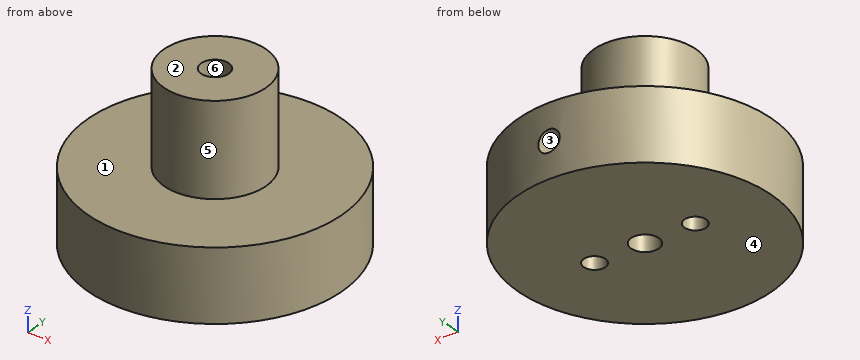
```python
from build123d import *

# Parameters (mm, degrees)
SKETCH1_R                 = 15.8115
BOSS_EXTRUDE1_DEPTH       = 25.4
SKETCH2_OUTSIDE_W         = 43.91
SKETCH2_OUTSIDE_H         = 43.91
SKETCH2_OUTSIDE_R         = 6.35
CUT_EXTRUDE1_DEPTH        = 16.51
F_8_32_TAPPED_HOLE1_D     = 3.4544
F_6_32_TAPPED_HOLE2_D     = 2.7051
F_6_32_TAPPED_HOLE2_DEPTH = 6.858
F_6_32_TAPPED_HOLE2_TIP   = 0.81269403
F_6_32_TAPPED_HOLE3_D     = 2.7051
F_6_32_TAPPED_HOLE3_DEPTH = 6.096
F_6_32_TAPPED_HOLE3_TIP   = 0.81269403
SKETCH9_R                 = 6.35
CUT_EXTRUDE3_DEPTH        = 5.08


with BuildPart() as part:
    # Sketch1 → Boss-Extrude1 (new body)
    with BuildSketch(Plane.XY):
        Circle(SKETCH1_R)
    extrude(amount=BOSS_EXTRUDE1_DEPTH)

    # Sketch2 outside → Cut-Extrude1 (cut)
    with BuildSketch(Plane.XY.offset(25.4)):
        Rectangle(SKETCH2_OUTSIDE_W, SKETCH2_OUTSIDE_H)
        Circle(SKETCH2_OUTSIDE_R, mode=Mode.SUBTRACT)
    extrude(amount=-CUT_EXTRUDE1_DEPTH, mode=Mode.SUBTRACT)

    # #8-32 Tapped Hole1 (through all)
    with Locations(Plane.XY.offset(25.4)):
        with Locations((0, 0)):
            Hole(F_8_32_TAPPED_HOLE1_D / 2)

    # #6-32 Tapped Hole2
    with Locations(Plane(origin=(0, 0, 0), x_dir=(-1, 0, 0), z_dir=(0, 0, -1))):
        with Locations((-6.35, 0), (6.35, 0)):
            Hole(F_6_32_TAPPED_HOLE2_D / 2, depth=F_6_32_TAPPED_HOLE2_DEPTH)
            with Locations((0, 0, -(F_6_32_TAPPED_HOLE2_DEPTH + F_6_32_TAPPED_HOLE2_TIP / 2))):  # 118° drill point
                Cone(0, F_6_32_TAPPED_HOLE2_D / 2, F_6_32_TAPPED_HOLE2_TIP, mode=Mode.SUBTRACT)

    # #6-32 Tapped Hole3
    with Locations(Plane(origin=(0, 15.8115, 4.445), x_dir=(1, 0, 0), z_dir=(0, 1, 0))):
        with Locations((0, 0)):
            Hole(F_6_32_TAPPED_HOLE3_D / 2, depth=F_6_32_TAPPED_HOLE3_DEPTH)
            with Locations((0, 0, -(F_6_32_TAPPED_HOLE3_DEPTH + F_6_32_TAPPED_HOLE3_TIP / 2))):  # 118° drill point
                Cone(0, F_6_32_TAPPED_HOLE3_D / 2, F_6_32_TAPPED_HOLE3_TIP, mode=Mode.SUBTRACT)

    # Sketch9 → Cut-Extrude3 (cut)
    with BuildSketch(Plane.XY.offset(25.4)):
        Circle(SKETCH9_R)
    extrude(amount=-CUT_EXTRUDE3_DEPTH, mode=Mode.SUBTRACT)


solid = part.part
```
For this review, take the finished solid that the model builds, in its own axes (mm). Face numbers are marked on the shaded views. A direction names the side the tool comes from. Coordinates: 2 decimals unless noted, no trailing zeros. Loops run counter-clockwise (first coordinate to the right, second up) from the corner with the lowest first, then second, coordinate; pieces in that order, holes last. Notation, with made-up numbers: (25.5, 0.5) - (46.5, 0.5) arc R8 cw to (46.5, 14.5) - close; hole circle Ø1 at (72, 46.5). An arc over 180 degrees is marked (long way). Use one line per item in the form item = value. Start each with the question number.
1) For the marked faces 1, 2 and 3, list the 3-axis set-ups (+Z, -Z, +X, -X, +Y, -Y) from which the entire face can be reached by the end or side of a thin tool; tool diameter is ignored.
2) Take a section at A-A (z = 1.5). State the section outline as (x, y) points.
3) Take a section at B-B (x = 4). State the section outline as (y, z) points, plus the area to 3 significant figures.
4) Draft analysis for pull direction X (two halves, no side actions). For the marked faces 4, 5 and 6, state which applies: released by +X, released by -X, zero draft, split by the parting line, or undercut.
5) To check wall thickness, follow probe 1 along Y at (x, z) = (0, 9.25); probe 2 along Z at (x, y) = (0, 13.5); probe 3 along Z at (x, y) = (14, -1). State the ranges of each line that lie inside material, in increasing order. Write a range as from..to.
6) Take a section at D-D (z = 12). State the section outline as (x, y) points, plus the area to 3 significant figures.
7) For pin 1 (12 mm diameter, centred on y = -10, z = 16.5, fed in from -X); pin 2 (1.5 mm diameter, centred on x = 6.5, z = 17, fed in from +Y); pin 3 (3 mm diameter, centred on x = -8, y = 0.5, fed in from +Z), all flat-tipped, find the tip position at first contact; note any pin that passes through.
From the geometry:
q1.face_1 = +Z
q1.face_2 = +Z, +X, -X, +Y, -Y
q1.face_3 = +Y
q2.outline = circle Ø31.62 at (0, 0); hole circle Ø2.71 at (-6.35, 0); hole circle Ø3.45 at (0, 0); hole circle Ø2.71 at (6.35, 0)
q3.outline = (-15.3, 0) - (15.3, 0) - (15.3, 8.89) - (4.93, 8.89) - (4.93, 20.32) - (-4.93, 20.32) - (-4.93, 8.89) - (-15.3, 8.89) - close
q3.area = 385 mm2
q4.face_4 = zero draft
q4.face_5 = split by the parting line
q4.face_6 = undercut
q5.probe_1 = -6.35..-1.73, 1.73..6.35
q5.probe_2 = 0..3.09, 5.8..8.89
q5.probe_3 = 0..8.89
q6.outline = circle Ø12.7 at (0, 0); hole circle Ø3.45 at (0, 0)
q6.area = 117 mm2
q7.pin_1 = -4.93
q7.pin_2 = 2.69
q7.pin_3 = 8.89
